Verification items for this drawing (mm, ordinates from the low corner). A direction names the side the tool comes from. Round coordinates to 2 decimals unless told otherwise and drop trailing zeros. Order: outer loops, then holes, each group sorted by start corner. A loop starts at its lowest first (then second) coordinate and runs counter-clockwise, first axis right, second up. Notation, with made-up numbers: M 81,59 L 111,59 A21 ccw 111,68 Z; hole C -20,-30 d11. An arc over 180 degrees is marked long. One line per item, written item: value. Start each with the question number.
(1) Cross-section at C-C, the plane y = 6.35. Enter the section's corners in (x, z).
(2) Cross-section at A-A, the plane y = 10.7. Enter the section's corners in (x, z), and give its area (3 significant figures).
(3) Cross-section at D-D, the plane z = 9.75. Enter the section's corners in (x, y).
(4) Access from +Z, -Z, +X, -X, +Y, -Y to the whole of each face (thin tool, end or side, straight path). Record for the marked faces 4, 5 and 6.
(5) Release check for a two-part mould opening along X. For the marked faces 1, 2 and 3 record: released by +X, released by -X, zero draft, split by the parting line, or undercut.
(6) Thickness scan on L1, parallel to Y at x = 10.7, z = 5.45; L2, parallel to Y at x = 6.5, z = 8; L3, parallel to Z at x = 8.5, y = 7.25. Record the ranges inside material, lowest first.
(7) Depth check by flat-ended pin: pin 1 Ø3 at (x, y) = (2, 10.7) entering from +Z; pin 2 Ø2 at (y, z) = (6.5, 3.5) entering from -X; pin 3 Ø4 at (x, y) = (10.7, 2) entering from -Z; pin 4 Ø1 at (x, y) = (2, 1.5) entering from -Z. Enter the tip coordinate at first touch or a pass-through.
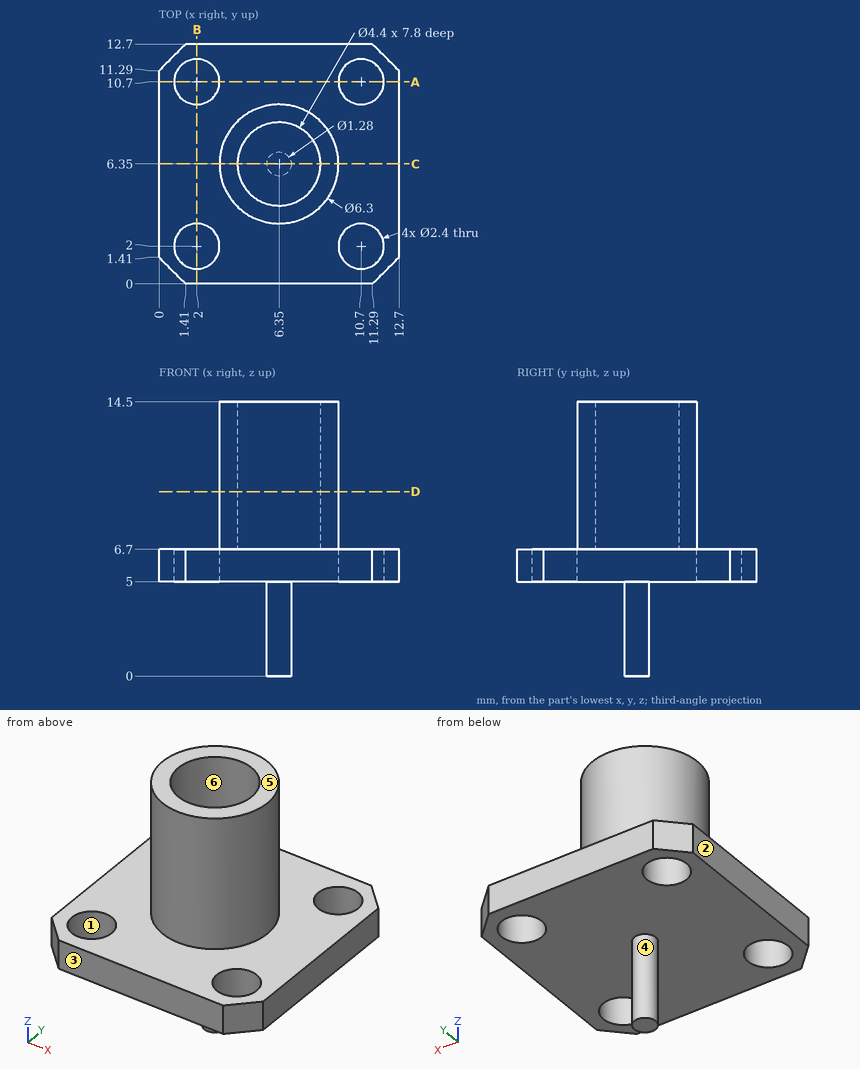
Values found:
1. outline: M 0,5 L 5.71,5 L 5.71,0 L 6.99,0 L 6.99,5 L 12.7,5 L 12.7,6.7 L 9.5,6.7 L 9.5,14.5 L 8.55,14.5 L 8.55,6.7 L 4.15,6.7 L 4.15,14.5 L 3.2,14.5 L 3.2,6.7 L 0,6.7 Z
2. outline: M 0,5 L 0.8,5 L 0.8,6.7 L 0,6.7 Z; M 3.2,5 L 9.5,5 L 9.5,6.7 L 3.2,6.7 Z; M 11.9,5 L 12.7,5 L 12.7,6.7 L 11.9,6.7 Z
2. area: 13.4 mm^2
3. outline: C 6.35,6.35 d6.3; hole C 6.35,6.35 d4.4
4. face 4: -Z
4. face 5: +Z, +X, -X, +Y, -Y
4. face 6: +Z
5. face 1: undercut
5. face 2: released by -X
5. face 3: zero draft
6. L1: 0 to 0.8, 3.2 to 9.5, 11.9 to 12.7
6. L2: 3.2 to 4.16, 8.54 to 9.5
6. L3: 5 to 14.5
7. pin 1: z = 6.7
7. pin 2: x = 5.71
7. pin 3: z = 5
7. pin 4: through
